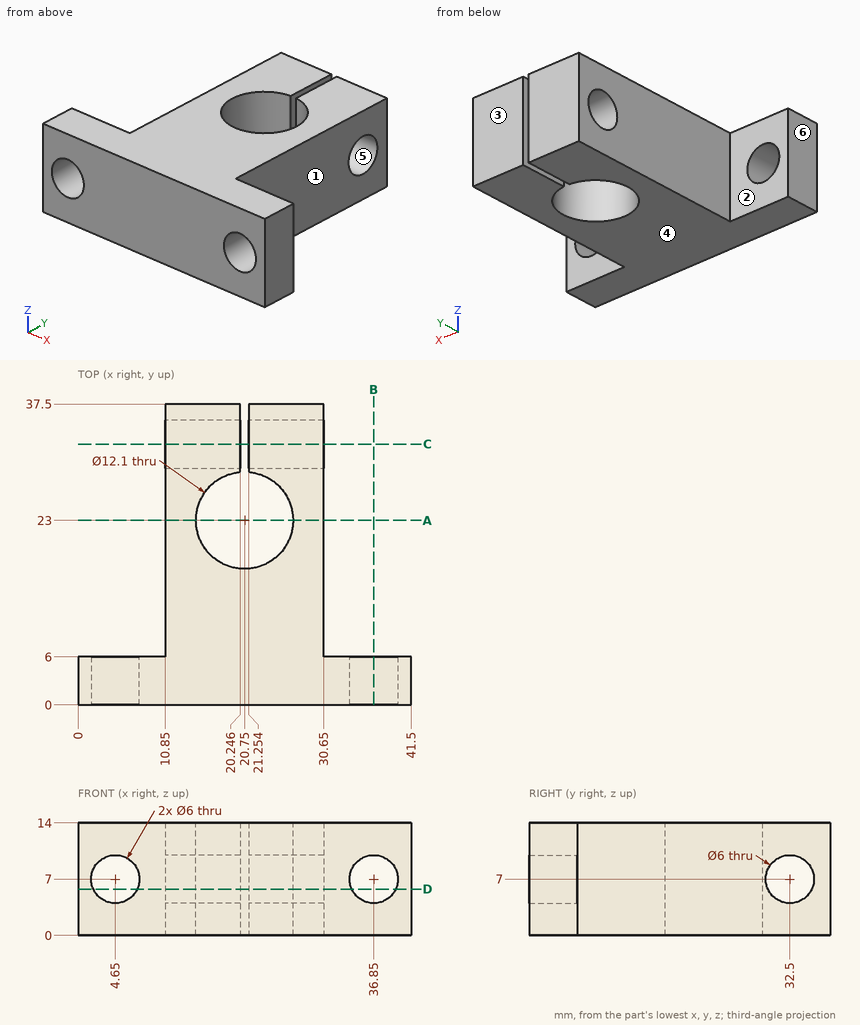
Input: dimensioned drawing with shaded views. Units: mm. Origin: part minimum x, y, z. A direction names the side the tool comes from. Give positions to 0.01 mm unless a question says otherwise; leave off trailing zeros. Order: outer loops, then holes, each group sorted by start corner. A loop starts at its lowest first (then second) coordinate and runs counter-clockwise, first axis right, second up. Notation, with made-up numbers: (88.5, 68) -> (117.5, 68) arc R25 ccw to (117.5, 92) -> close; hole circle Ø1 at (35.5, 84.25). An arc over 180 degrees is marked (long way). Use one line per item in the form item = value.
1) Section C-C, the plane y = 32.5. Return loops of the section in (x, z), and give its area (3 significant figures).
Response values:
outline = (10.85, 0) -> (20.25, 0) -> (20.25, 4) -> (10.85, 4) -> close; (10.85, 10) -> (20.25, 10) -> (20.25, 14) -> (10.85, 14) -> close; (21.25, 0) -> (30.65, 0) -> (30.65, 4) -> (21.25, 4) -> close; (21.25, 10) -> (30.65, 10) -> (30.65, 14) -> (21.25, 14) -> close
area = 150 mm^2
2) Section D-D, the plane z = 5.75. Return loops of the section in (x, y).
Response values:
outline = (0, 0) -> (1.92, 0) -> (1.92, 6) -> (0, 6) -> close; (7.38, 0) -> (34.12, 0) -> (34.12, 6) -> (30.65, 6) -> (30.65, 29.77) -> (21.25, 29.77) -> (21.25, 29.03) arc R6.05 cw (long way) to (20.25, 29.03) -> (20.25, 29.77) -> (10.85, 29.77) -> (10.85, 6) -> (7.38, 6) -> close; (10.85, 35.23) -> (20.25, 35.23) -> (20.25, 37.5) -> (10.85, 37.5) -> close; (21.25, 35.23) -> (30.65, 35.23) -> (30.65, 37.5) -> (21.25, 37.5) -> close; (39.58, 0) -> (41.5, 0) -> (41.5, 6) -> (39.58, 6) -> close
3) First-contact query: pin 1 Ø1.5 at (y, z) = (11.5, 11) entering from -X; pin 2 Ø2.5 at (y, z) = (33, 4.5) entering from +X; pin 3 Ø7.5 at (x, y) = (20.75, 23) entering from +Z; pin 4 Ø5.5 at (x, z) = (37.5, 5.5) entering from +Y. Flat tips, straight axial feed; report the tip coordinate or a pass-through.
Response values:
pin_1 = 10.85
pin_2 = 30.65
pin_3 = through
pin_4 = 6
4) Section A-A, the plane y = 23. Return loops of the section in (x, z).
Response values:
outline = (10.85, 0) -> (14.7, 0) -> (14.7, 14) -> (10.85, 14) -> close; (26.8, 0) -> (30.65, 0) -> (30.65, 14) -> (26.8, 14) -> close
5) Mould query, pull axis Z, two halves, no side actions, for the marked faces 4, 5 and 6. Classes: pulls with the +Z half, pulls with the -Z half, needs draft (parallel to the pull), parting line crosses it, or undercut.
Response values:
face_4 = pulls with the -Z half
face_5 = undercut
face_6 = needs draft
6) Reachability of the marked faces 1, 2 and 3 from +Z, -Z, +X, -X, +Y, -Y: full face, straight path, thin tool, end or side. Return the list, or none.
Response values:
face_1 = +Z, -Z, +X, +Y
face_2 = +Z, -Z, -X, +Y
face_3 = +Z, -Z, +X, -X, +Y
7) Line query: probe 1 along Z at (x, y) = (36.85, 4.25); probe 2 along Y at (x, z) = (17.5, 6.25) (1 decimal); probe 3 along X at (y, z) = (5.5, 8.75). Output: solid intervals per line, ascending.
Response values:
probe_1 = 0 to 4, 10 to 14
probe_2 = 0 to 17.9, 28.1 to 29.6, 35.4 to 37.5
probe_3 = 0 to 2.21, 7.09 to 34.41, 39.29 to 41.5
8) Section B-B, the plane x = 36.85. Return loops of the section in (y, z), and give its area (3 significant figures).
Response values:
outline = (0, 0) -> (6, 0) -> (6, 4) -> (0, 4) -> close; (0, 10) -> (6, 10) -> (6, 14) -> (0, 14) -> close
area = 48.0 mm^2
